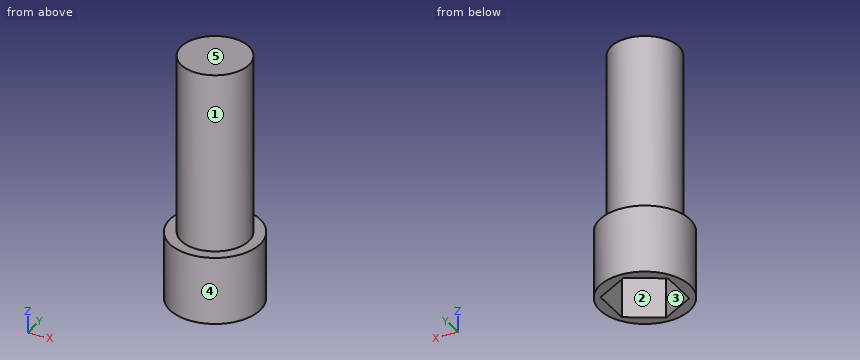
from build123d import *

# Parameters (mm, degrees)
SKETCH_1_R          = 2
EXTRUDE_1_DEPTH     = 3
SKETCH_2_R          = 1.5
EXTRUDE_2_DEPTH     = 8
CUT_EXTRUDE_1_DEPTH = 2


with BuildPart() as part:
    # 草图1 → 凸台-拉伸1 (new body)
    with BuildSketch(Plane.XY):
        Circle(SKETCH_1_R)
    extrude(amount=EXTRUDE_1_DEPTH)

    # 草图2 → 凸台-拉伸2 (add)
    with BuildSketch(Plane.XY.offset(3)):
        Circle(SKETCH_2_R)
    extrude(amount=EXTRUDE_2_DEPTH)

    # 草图3 → 切除-拉伸1 (cut)
    with BuildSketch(Plane(origin=(0, 0, 0), x_dir=(-1, 0, 0), z_dir=(0, 0, -1))):
        Polygon((1.513862997, -0.841557381), (1.485741569, 0.890265123), (-0.028121428, 1.731822504), (-1.513862997, 0.841557381), (-1.485741569, -0.890265123), (0.028121428, -1.731822504), align=None)
    extrude(amount=-CUT_EXTRUDE_1_DEPTH, mode=Mode.SUBTRACT)


solid = part.part
Geometry: final body of the model. Coordinates: model frame, mm. Face numbers are marked on the shaded views. A direction names the side the tool comes from. Coordinates: 2 decimals unless noted, no trailing zeros. Order: outer loops, then holes, each group sorted by start corner. A loop starts at its lowest first (then second) coordinate and runs counter-clockwise, first axis right, second up. Notation, with made-up numbers: (68, 10.5) - (116, 10.5) arc R38 cw to (116, 49.5) - close; hole circle Ø4 at (74.5, -6). An arc over 180 degrees is marked (long way). Use one line per item in the form item = value.
1) Mould query, pull axis Y, two halves, no side actions, for the marked faces 3, 4 and 5. Classes: +Y half, -Y half, draft (parallel to the pull), parting line (faces both ways), or undercut.
Solutions:
face_3 = undercut
face_4 = parting line
face_5 = draft
2) Section A-A (y = 1.25). Return loops of the section in (x, z).
Solutions:
outline = (-1.56, 0) - (-0.84, 0) - (-0.84, 2) - (0.83, 2) - (0.83, 0) - (1.56, 0) - (1.56, 3) - (0.83, 3) - (0.83, 11) - (-0.83, 11) - (-0.83, 3) - (-1.56, 3) - close
3) Section C-C (z = 10.5). Return loops of the section in (x, y).
Solutions:
outline = circle Ø3 at (0, 0)
4) Section D-D (x = -1.65). Return loops of the section in (y, z), then the cut area to 3 significant figures.
Solutions:
outline = (-1.13, 0) - (1.13, 0) - (1.13, 3) - (-1.13, 3) - close
area = 6.78 mm^2
5) Pin query (flat end, axial travel): pin 1 (1.5 mm diameter, centred on x = -0.5, y = 0, fed in from -Z); pin 2 (2 mm diameter, centred on x = -1.5, z = 2, fed in from -Y); pin 3 (2 mm diameter, centred on y = -1, z = 8, fed in from -X). Return the tip coordinate at first contact, or that it passes through.
Solutions:
pin_1 = 2
pin_2 = -1.94
pin_3 = -1.5
6) Set-up query: the marked faces 1 and 2. Return all of +Z, -Z, +X, -X, +Y, -Y with unobstructed straight access to the full face (end or side cutting, diameter ignored); none if empty.
Solutions:
face_1 = +Z
face_2 = -Z
7) Ray query, L1, parallel to Z at x = 0.9, y = -1.5; L2, parallel to Z at x = -1.15, y = 1; L3, parallel to X at y = 0.45, z = 1. Return the intervals inside material, ascending.
Solutions:
L1 = 0 to 3
L2 = 2 to 3
L3 = -1.95 to -1.49, 1.51 to 1.95
8) Section B-B (x = 0.4). Return loops of the section in (y, z), then the cut area to 3 significant figures.
Solutions:
outline = (-1.96, 0) - (-1.49, 0) - (-1.49, 2) - (1.51, 2) - (1.51, 0) - (1.96, 0) - (1.96, 3) - (1.45, 3) - (1.45, 11) - (-1.45, 11) - (-1.45, 3) - (-1.96, 3) - close
area = 28.9 mm^2
